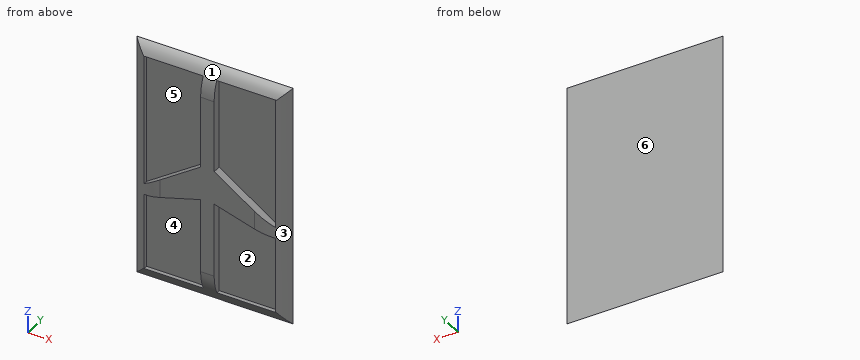
from build123d import *

# Parameters (mm, degrees)
F1_DEPTH    = 6
F0_W        = 76.4068576
F0_H        = 116.405787
F2_DEPTH    = 6
F3_DEPTH    = 2
F4_T1_DEPTH = 192.098587186
F4_T3_DEPTH = 152.099657786


# Not quite as in the source:
# - a fillet or chamfer that OpenCascade refuses, or shapes differently, is made with other operations: its cross-section is extruded or revolved along the edge and cut away or added
# - a feature names something its author has since deleted; it is built from what else it names


with BuildPart() as f1:
    # F0 (on Front) → F1 (new body)
    with BuildSketch(Plane.XZ):
        Polygon((15.6125306649, 37.6914590597), (9.0085306649, 37.6914590597), (9.0085306649, -6.1789248552), (-19.818228389, -25.1597724855), (-19.818228389, -30.4937724855), (9.0085306649, -22.2596581395), (9.0085306649, -67.1633433111), (15.6125306649, -67.1633433111), (15.6125306649, -22.2596581395), (44.4392897189, -30.4937724855), (44.4392897189, -25.1597724855), (15.6125306649, -6.1789248552), align=None)
    extrude(amount=F1_DEPTH)

    # F0 (on Front) → F2 (join)
    with BuildSketch(Plane.XZ):
        with Locations((12.3105306649, -14.7359421257)):
            Rectangle(F0_W, F0_H)
        Polygon((-19.818228389, -25.1597724855), (-19.818228389, 37.6914590597), (9.0085306649, 37.6914590597), (15.6125306649, 37.6914590597), (44.4392897189, 37.6914590597), (44.4392897189, -25.1597724855), (44.4392897189, -30.4937724855), (44.4392897189, -67.1633433111), (15.6125306649, -67.1633433111), (9.0085306649, -67.1633433111), (-19.818228389, -67.1633433111), (-19.818228389, -30.4937724855), align=None, mode=Mode.SUBTRACT)
    extrude(amount=F2_DEPTH)

    # F0 (on Front) → F3 (join)
    with BuildSketch(Plane.XZ):
        Polygon((9.0085306649, 37.6914590597), (-19.818228389, 37.6914590597), (-19.818228389, -25.1597724855), (9.0085306649, -6.1789248552), align=None)
        Polygon((44.4392897189, -67.1633433111), (44.4392897189, -30.4937724855), (15.6125306649, -22.2596581395), (15.6125306649, -67.1633433111), align=None)
        Polygon((9.0085306649, -22.2596581395), (-19.818228389, -30.4937724855), (-19.818228389, -67.1633433111), (9.0085306649, -67.1633433111), align=None)
        Polygon((44.4392897189, 37.6914590597), (15.6125306649, 37.6914590597), (15.6125306649, -6.1789248552), (44.4392897189, -25.1597724855), align=None)
    extrude(amount=F3_DEPTH)

    # F4: fillet of radius 22.098 on 4 edges, made by hand

    # F4_s2 → F4_t1 (cut)
    with BuildSketch(Plane.XY.offset(-110.7852357187)):
        with BuildLine():
            ThreePointArc((-25.8928981351, 0), (-18.8964508458, -4.445310444), (-10.7543380979, -6))
            Line((-10.7543380979, -6), (-25.8928981351, -6))
            Line((-25.8928981351, -6), (-25.8928981351, 0))
        make_face()
        with BuildLine():
            ThreePointArc((50.5139594649, 0), (43.5175121757, -4.445310444), (35.3753994277, -6))
            Line((35.3753994277, -6), (50.5139594649, -6))
            Line((50.5139594649, -6), (50.5139594649, 0))
        make_face()
    extrude(amount=F4_T1_DEPTH, mode=Mode.SUBTRACT)

    # F4_s4 → F4_t3 (cut)
    with BuildSketch(Plane.YZ.offset(-63.7392982281)):
        with BuildLine():
            ThreePointArc((0, -72.9388356257), (-4.445310444, -65.9423883364), (-6, -57.8002755885))
            Line((-6, -57.8002755885), (-6, -72.9388356257))
            Line((-6, -72.9388356257), (0, -72.9388356257))
        make_face()
        with BuildLine():
            ThreePointArc((-6, 28.3283913371), (-4.445310444, 36.4705040851), (0, 43.4669513743))
            Line((0, 43.4669513743), (-6, 43.4669513743))
            Line((-6, 43.4669513743), (-6, 28.3283913371))
        make_face()
    extrude(amount=F4_T3_DEPTH, mode=Mode.SUBTRACT)


solid = f1.part
Geometry check sheet. Reference: the model listing, model coordinates, mm. Face numbers are marked on the shaded views. A direction names the side the tool comes from. Give positions to 0.01 mm unless a question says otherwise; leave off trailing zeros. Order: outer loops, then holes, each group sorted by start corner. A loop starts at its lowest first (then second) coordinate and runs counter-clockwise, first axis right, second up.
1. Access from +Z, -Z, +X, -X, +Y, -Y to the whole of each face (thin tool, end or side, straight path). Record for the marked faces 5 and 6.
Completed:
face 5: -Y
face 6: +Z, -Z, +X, -X, +Y
2. Depth check by flat-ended pin: pin 1 (1 mm diameter, centred on y = -2.5, z = 13.5, fed in from +X); pin 2 (0.6 mm diameter, centred on y = -3, z = -54, fed in from +X); pin 3 (2 mm diameter, centred on x = 14, y = -2, fed in from -Z). Enter the tip coordinate at first touch or a pass-through.
Completed:
pin 1: stops at x = 48.06
pin 2: stops at x = 46.99
pin 3: stops at z = -71.8
3. Sectioned sample at A-A (z = -45.5). Record the boundary of the cut face in (x, y).
Completed:
outline: (-25.89, 0) arc R22.1 ccw to (-19.82, -4.06) - (-19.82, -2) - (9.01, -2) - (9.01, -6) - (15.61, -6) - (15.61, -2) - (44.44, -2) - (44.44, -4.06) arc R22.1 ccw to (50.51, 0) - close
4. Draft check along X on the marked faces 1, 2, 3 and 4. Enter one of: pulls with the +X half, pulls with the -X half, needs draft (parallel to the pull), parting line crosses it, or undercut.
Completed:
face 1: needs draft
face 2: undercut
face 3: pulls with the +X half
face 4: undercut
5. Sectioned sample at C-C (x = -7.5). Record the boundary of the cut face in (y, z), then the cut area to 3 significant figures.
Completed:
outline: (-6, -26.98) - (-2, -26.98) - (-2, -67.16) - (-3.92, -67.16) arc R22.1 ccw to (0, -72.94) - (0, 43.47) arc R22.1 ccw to (-3.92, 37.69) - (-2, 37.69) - (-2, -17.05) - (-6, -17.05) - close
area: 275 mm2
6. Scan lines: line 1 (Z direction, x = 0.5, y = -2.25); line 2 (X direction, y = -2.5, z = -38); line 3 (X direction, y = -3.5, z = 15). Record each from-to range of solid material in increasing order.
Completed:
line 1: z = -70.12 to -67.16, -24.69 to -11.78, 37.69 to 40.64
line 2: x = -22.69 to -19.82, 9.01 to 15.61, 44.44 to 47.31
line 3: x = -20.96 to -19.82, 9.01 to 15.61, 44.44 to 45.59
7. Sectioned sample at D-D (z = -21). Record the boundary of the cut face in (x, y), then the cut area to 3 significant figures.
Completed:
outline: (-25.89, 0) arc R22.1 ccw to (-19.82, -4.06) - (-19.82, -2) - (-13.5, -2) - (-13.5, -5.83) arc R22.1 ccw to (-10.75, -6) - (35.38, -6) arc R22.1 ccw to (38.12, -5.83) - (38.12, -2) - (44.44, -2) - (44.44, -4.06) arc R22.1 ccw to (50.51, 0) - close
area: 362 mm2
8. Sectioned sample at B-B (y = -3). Record the boundary of the cut face in (x, z).
Completed:
outline: (-21.87, -68.92) - (46.49, -68.92) - (46.49, 39.45) - (-21.87, 39.45) - close; hole (-19.82, -67.16) - (9.01, -67.16) - (9.01, -22.26) - (-19.82, -30.49) - close; hole (-19.82, -25.16) - (9.01, -6.18) - (9.01, 37.69) - (-19.82, 37.69) - close; hole (15.61, -67.16) - (44.44, -67.16) - (44.44, -30.49) - (15.61, -22.26) - close; hole (15.61, -6.18) - (44.44, -25.16) - (44.44, 37.69) - (15.61, 37.69) - close
